Part model, mm, in its own coordinate system. Round coordinates to 2 decimals unless told otherwise and drop trailing zeros. Loops run counter-clockwise (first coordinate to the right, second up) from the corner with the lowest first, then second, coordinate; pieces in that order, holes last.
from build123d import *

# Parameters (mm, degrees)
SKETCH1_R            = 39
SKETCH1_R_2          = 26.5
BOSS_EXTRUDE1_DEPTH  = 1.5
SKETCH3_W            = 50
SKETCH3_H            = 51.5
BOSS_EXTRUDE2_DEPTH  = 1.5
BOSS_EXTRUDE4_DEPTH  = 1.5
SKETCH2_R            = 2.75
CUT_EXTRUDE1_DEPTH   = 2.5
CIRPATTERN1_COUNT    = 6
CUT_EXTRUDE2_START   = -4
SKETCH5_R            = 2.25
CUT_EXTRUDE2_DEPTH   = 5
LPATTERN1_COUNT      = 2
LPATTERN1_PITCH      = 15
LPATTERN1_COUNT_DIR2 = 2
LPATTERN1_PITCH_DIR2 = 10
LPATTERN2_COUNT      = 2
LPATTERN2_PITCH      = 15
LPATTERN2_COUNT_DIR2 = 2
LPATTERN2_PITCH_DIR2 = 10
CUT_EXTRUDE3_START   = -4
SKETCH7_R            = 3.25
CUT_EXTRUDE3_DEPTH   = 5
LPATTERN3_COUNT      = 3
LPATTERN3_PITCH      = 20
SKETCH8_R            = 3.25
CUT_EXTRUDE4_DEPTH   = 10
LPATTERN4_COUNT      = 4
LPATTERN4_PITCH      = 20


with BuildPart() as part:
    # Sketch1 → Boss-Extrude1 (new body, symmetric)
    with BuildSketch(Plane(origin=(0, 0, 0), x_dir=(1, 0, 0), z_dir=(0, 1, 0))):
        Circle(SKETCH1_R)
        Circle(SKETCH1_R_2, mode=Mode.SUBTRACT)
    extrude(amount=BOSS_EXTRUDE1_DEPTH, both=True)

    # Sketch3 → Boss-Extrude2 (add, symmetric)
    with BuildSketch(Plane(origin=(0, 0, 0), x_dir=(1, 0, 0), z_dir=(0, 1, 0))):
        with Locations((0, 52.25)):
            Rectangle(SKETCH3_W, SKETCH3_H)
    extrude(amount=BOSS_EXTRUDE2_DEPTH, both=True)

    # Sketch6 → Boss-Extrude4 (add, symmetric)
    with BuildSketch(Plane(origin=(0, 0, 0), x_dir=(1, 0, 0), z_dir=(0, 1, 0))):
        Polygon((-35, 166.5), (-35, 26.5), (-39, 0), (-14.981514186, 26.5), (16.520833333, 26.5), (39, 0), (35, 26.5), (35, 166.5), align=None)
    extrude(amount=BOSS_EXTRUDE4_DEPTH, both=True)

    # Sketch2 → Cut-Extrude1 (cut, symmetric)
    with BuildSketch(Plane(origin=(0, 0, 0), x_dir=(1, 0, 0), z_dir=(0, 1, 0))):
        with Locations((0, 32.5)):
            Circle(SKETCH2_R)
    cut_extrude1 = extrude(amount=CUT_EXTRUDE1_DEPTH, both=True, mode=Mode.SUBTRACT)

    # CirPattern1: Cut-Extrude1 ×6 about axis
    cirpattern1_axis = Axis((0, 0, 0), (0, 1, 0))
    for i in range(1, CIRPATTERN1_COUNT):
        add(cut_extrude1.rotate(cirpattern1_axis, i * 360 / CIRPATTERN1_COUNT), mode=Mode.SUBTRACT)

    # Sketch5 → Cut-Extrude2 (cut)
    with BuildSketch(Plane(origin=(0, 1.5, 0), x_dir=(1, 0, 0), z_dir=(0, 1, 0)).offset(CUT_EXTRUDE2_START)):
        with Locations((0, 73)):
            Circle(SKETCH5_R)
    cut_extrude2 = extrude(amount=CUT_EXTRUDE2_DEPTH, mode=Mode.SUBTRACT)

    # LPattern1: Cut-Extrude2 2 × 2
    with Locations(*[(i * LPATTERN1_PITCH, 0, j * LPATTERN1_PITCH_DIR2) for i in range(LPATTERN1_COUNT) for j in range(LPATTERN1_COUNT_DIR2) if (i, j) != (0, 0)]):
        add(cut_extrude2, mode=Mode.SUBTRACT)

    # LPattern2: Cut-Extrude2 2 × 2
    with Locations(*[(-i * LPATTERN2_PITCH, 0, j * LPATTERN2_PITCH_DIR2) for i in range(LPATTERN2_COUNT) for j in range(LPATTERN2_COUNT_DIR2) if (i, j) != (0, 0)]):
        add(cut_extrude2, mode=Mode.SUBTRACT)

    # Sketch7 → Cut-Extrude3 (cut)
    with BuildSketch(Plane(origin=(0, 1.5, 0), x_dir=(1, 0, 0), z_dir=(0, 1, 0)).offset(CUT_EXTRUDE3_START)):
        with Locations((-15, 146.5)):
            Circle(SKETCH7_R)
        with Locations((15, 146.5)):
            Circle(SKETCH7_R)
    cut_extrude3 = extrude(amount=CUT_EXTRUDE3_DEPTH, mode=Mode.SUBTRACT)

    # LPattern3: Cut-Extrude3 ×3
    with Locations(*[(0, 0, i * LPATTERN3_PITCH) for i in range(1, LPATTERN3_COUNT)]):
        add(cut_extrude3, mode=Mode.SUBTRACT)

    # Sketch8 → Cut-Extrude4 (cut)
    with BuildSketch(Plane(origin=(0, 1.5, 0), x_dir=(1, 0, 0), z_dir=(0, 1, 0))):
        with Locations((0, 146.5)):
            Circle(SKETCH8_R)
    cut_extrude4 = extrude(amount=-CUT_EXTRUDE4_DEPTH, mode=Mode.SUBTRACT)

    # LPattern4: Cut-Extrude4 ×4
    with Locations(*[(0, 0, i * LPATTERN4_PITCH) for i in range(1, LPATTERN4_COUNT)]):
        add(cut_extrude4, mode=Mode.SUBTRACT)


solid = part.part
1) Slice it at C-C, the plane x = -7.5. Give the cut face in (y, z), then the cut area to 3 significant figures.
Values:
outline: (-1.5, -166.5) - (1.5, -166.5) - (1.5, -25.42) - (-1.5, -25.42) - close; (-1.5, 25.42) - (1.5, 25.42) - (1.5, 38.27) - (-1.5, 38.27) - close
area: 462 mm2
2) Mould opens along X. For faces 1 (the face through (16.5, -0.021, -143.617)), 2 (the face through (14.512, -0.021, -60.804)), 3 (the face through (8, 1.5, -65)), 4 (the face through (-1.021, 0.021, 38.987)) say: released by +X, released by -X, zero draft, split by the parting line, or undercut.
Values:
face 1: undercut
face 2: undercut
face 3: zero draft
face 4: split by the parting line
3) Drop flat-ended pins along their axis: pin 1 Ø4 at (x, z) = (0, -86.5) entering from -Y; pin 2 Ø7.5 at (x, z) = (0, -106.5) entering from -Y; pin 3 Ø1.5 at (x, y) = (-9, 0.5) entering from +Z; pin 4 Ø1.5 at (y, z) = (1, -35.5) entering from +X. Give the stop position or say it passes through.
Values:
pin 1: passes through
pin 2: stops at y = -1.5
pin 3: stops at z = 38.12
pin 4: stops at x = 35
4) Slice it at A-A, the plane z = 0. Give the cut face in (x, y).
Values:
outline: (-39, -1.5) - (-26.5, -1.5) - (-26.5, 1.5) - (-39, 1.5) - close; (26.5, -1.5) - (39, -1.5) - (39, 1.5) - (26.5, 1.5) - close
5) Wall check: line 1 along X through (y, z) = (0.1, -146.5); line 2 along Z through (x, y) = (-28, -0.25); line 3 along X through (y, z) = (-1.4, -80). Give the ranges that are in metal, low to high.
Values:
line 1: x = -35 to -18.25, -11.75 to -3.25, 3.25 to 11.75, 18.25 to 35
line 2: z = -166.5 to -19, -13.5 to 13.5, 19 to 27.15
line 3: x = -35 to 35
6) Slice it at D-D, the plane x = 15. Give the cut face in (y, z).
Values:
outline: (-1.5, -166.5) - (1.5, -166.5) - (1.5, -149.75) - (-1.5, -149.75) - close; (-1.5, -143.25) - (1.5, -143.25) - (1.5, -129.75) - (-1.5, -129.75) - close; (-1.5, -123.25) - (1.5, -123.25) - (1.5, -109.75) - (-1.5, -109.75) - close; (-1.5, -103.25) - (1.5, -103.25) - (1.5, -75.25) - (-1.5, -75.25) - close; (-1.5, -70.75) - (1.5, -70.75) - (1.5, -65.25) - (-1.5, -65.25) - close; (-1.5, -60.75) - (1.5, -60.75) - (1.5, -21.85) - (-1.5, -21.85) - close; (-1.5, 21.85) - (1.5, 21.85) - (1.5, 36) - (-1.5, 36) - close
7) Slice it at B-B, the plane z = -73. Give the cut face in (x, y), then the cut area to 4 significant figures.
Values:
outline: (-35, -1.5) - (-17.25, -1.5) - (-17.25, 1.5) - (-35, 1.5) - close; (-12.75, -1.5) - (-2.25, -1.5) - (-2.25, 1.5) - (-12.75, 1.5) - close; (2.25, -1.5) - (12.75, -1.5) - (12.75, 1.5) - (2.25, 1.5) - close; (17.25, -1.5) - (35, -1.5) - (35, 1.5) - (17.25, 1.5) - close
area: 169.5 mm2
